Source: CAD feature listing. Evaluate the final solid. Frame: model axes, mm. A direction names the side the tool comes from. Coordinates: 2 decimals unless noted, no trailing zeros. Order: outer loops, then holes, each group sorted by start corner. A loop starts at its lowest first (then second) coordinate and runs counter-clockwise, first axis right, second up. Notation, with made-up numbers: (53, 25.25) -> (71, 25.25) arc R17 ccw to (71, 53.25) -> close; hole circle Ø10 at (-24, 48.25). An arc over 180 degrees is marked (long way). Write each question's results on one line, items separated by ' | '. Start each with the question number.
from build123d import *

# Parameters (mm, degrees)
F1_DEPTH = 25.4
F3_DEPTH = 25.4
F5_DEPTH = 25.4
F6_R     = 5.646006
F6_R_2   = 5.670557
F7_DEPTH = 25.4


with BuildPart() as f1:
    # F0 (on Front) → F1 (new body)
    with BuildSketch(Plane.XZ):
        Polygon((0, 50.8), (0, 0), (57.15, 0), (57.15, 12.7), (12.7, 12.7), (12.7, 50.8), align=None)
    extrude(amount=F1_DEPTH)

    # F2 (on face) → F3 (cut)
    with BuildSketch(Plane.YZ.offset(12.7)):
        with BuildLine():
            ThreePointArc((-17.234911, 39.960572), (-12.701006, 35.423648), (-8.165089, 39.958559))
            ThreePointArc((-8.165089, 39.958559), (-8.16513, 39.977817), (-8.165252, 39.997075))
            ThreePointArc((-8.165252, 39.997075), (-12.718252, 44.493433), (-17.234911, 39.960572))
        make_face()
        with BuildLine():
            ThreePointArc((-25.4, 43.071147), (-21.877422, 47.527146), (-17.234911, 50.8))
            Line((-17.234911, 50.8), (-25.4, 50.8))
            Line((-25.4, 50.8), (-25.4, 43.071147))
        make_face()
        with BuildLine():
            ThreePointArc((-17.234911, 39.960572), (-12.718252, 44.493433), (-8.165252, 39.997075))
            Line((-8.165252, 39.997075), (-8.257007, 50.8))
            Line((-8.257007, 50.8), (-17.234911, 50.8))
            Line((-17.234911, 50.8), (-17.234911, 39.960572))
        make_face()
        with BuildLine():
            Line((0, 50.8), (-8.257007, 50.8))
            ThreePointArc((-8.257007, 50.8), (-3.471366, 47.637617), (0, 43.071147))
            Line((0, 43.071147), (0, 50.8))
        make_face()
    extrude(amount=-F3_DEPTH, mode=Mode.SUBTRACT)

    # F4 (on face) → F5 (cut)
    with BuildSketch(Plane.XY.offset(12.7)):
        with BuildLine():
            ThreePointArc((44.68115, 0), (52.530241, -4.764723), (57.15, -12.7))
            Line((57.15, -12.7), (57.15, 0))
            Line((57.15, 0), (44.68115, 0))
        make_face()
        with BuildLine():
            Line((57.15, -25.4), (57.15, -12.7))
            ThreePointArc((57.15, -12.7), (52.52777, -20.632851), (44.68115, -25.4))
            Line((44.68115, -25.4), (57.15, -25.4))
        make_face()
    extrude(amount=F5_DEPTH, mode=Mode.SUBTRACT)

    # F6 (on face) → F7 (cut)
    with BuildSketch(Plane.XY.offset(12.7)):
        with Locations((45.78362, -12.7)):
            Circle(F6_R)
        with Locations((30.217472, -12.7)):
            Circle(F6_R_2)
        with BuildLine():
            ThreePointArc((45.78362, 0), (53.145869, -4.847258), (57.15, -12.7))
            Line((57.15, -12.7), (57.15, 0))
            Line((57.15, 0), (45.78362, 0))
        make_face()
        with BuildLine():
            Line((57.15, -25.4), (57.15, -12.7))
            ThreePointArc((57.15, -12.7), (53.370398, -20.753693), (45.78362, -25.4))
            Line((45.78362, -25.4), (57.15, -25.4))
        make_face()
    extrude(amount=-F7_DEPTH, mode=Mode.SUBTRACT)


solid = f1.part
(1) Line query: L1, parallel to Z at x = 38, y = -21.75; L2, parallel to X at y = -7.5, z = 5. Output: solid intervals per line, ascending.
(2) Reachability of faces 1 (the cylindrical face through (53.454, -20.659, 6.439)), 2 (the flat face through (6, -17.235, 45)), 3 (the flat face through (35.24, -9.7, 12.7)) from +Z, -Z, +X, -X, +Y, -Y: full face, straight path, thin tool, end or side. Return the list, or none.
(3) Section D-D on z = 30. Return the cut outline in (x, y).
(4) Draft query along Y for faces 4 (the flat face through (0, -13, 20)), 5 (the cylindrical face through (53.06, -4.75, 6.44)), 6 (the flat face through (17, -25.4, 12)), 7 (the cylindrical face through (41.622, -8.884, 6.439)). Return one class per face: released by +Y, released by -Y, zero draft, split by the parting line, or undercut.
(5) Section C-C on z = 47. Return the cut outline in (x, y).
(6) Section B-B on x = 29. Return the cut outline in (y, z), then the cut area to 3 significant figures.
(7) First-contact query: P1, Ø3, axis at y = -15.5, z = 7.5, coming from the -X side; P2, Ø10, axis at x = 45.78, y = -12.7, coming from the +Z side; P3, Ø12, axis at x = 24, y = -7, coming from the +Z side; P4, Ø7.5, axis at y = -18.5, z = 33.5, coming from the +X side. Flat tips, straight axial feed; report the tip coordinate or a pass-through.
(8) Section A-A on y = -10.75. Return the cut outline in (x, z).
Results list:
1) L1: z = 0 to 12.7 | L2: x = 0 to 27.96, 32.48 to 43.58, 47.98 to 55.1
2) face 1: +Z, -Z, +X, -Y | face 2: +Z, +X, -X | face 3: +Z, +X, +Y, -Y
3) outline: (0, -25.4) -> (12.7, -25.4) -> (12.7, 0) -> (0, 0) -> close
4) face 4: zero draft | face 5: released by +Y | face 6: released by -Y | face 7: undercut
5) outline: (0, -22.41) -> (12.7, -22.41) -> (12.7, -17.23) -> (0, -17.23) -> close; (0, -8.22) -> (12.7, -8.22) -> (12.7, -2.83) -> (0, -2.83) -> close
6) outline: (-25.4, 0) -> (-18.24, 0) -> (-18.24, 12.7) -> (-25.4, 12.7) -> close; (-7.16, 0) -> (0, 0) -> (0, 12.7) -> (-7.16, 12.7) -> close | area: 182 mm²
7) P1: stops at x = 0 | P2: passes through | P3: stops at z = 12.7 | P4: stops at x = 12.7
8) outline: (0, 0) -> (24.89, 0) -> (24.89, 12.7) -> (12.7, 12.7) -> (12.7, 35.86) -> (0, 35.86) -> close; (35.54, 0) -> (40.49, 0) -> (40.49, 12.7) -> (35.54, 12.7) -> close; (51.08, 0) -> (56.61, 0) -> (56.61, 12.7) -> (51.08, 12.7) -> close
